The listing builds one solid part. Answer for the finished solid, in the listing's coordinates (mm). A direction names the side the tool comes from. Give positions to 0.01 mm unless a question says otherwise; leave off trailing zeros. Order: outer loops, then holes, each group sorted by start corner. A loop starts at its lowest first (then second) coordinate and runs counter-clockwise, first axis right, second up. Notation, with made-up numbers: (-12.5, -26) - (10.5, -26) arc R23 ccw to (10.5, 8) - close; hole circle Ø1 at (11.5, 17.25). An arc over 180 degrees is marked (long way). Use a Markdown table: item, result. Add a question column.
1) Find section C-C, the plane y = 0. Determine the outline of the cut face in (x, z).
2) Find section A-A, the plane x = -13.85. Determine the outline of the cut face in (y, z), plus the area to 3 significant figures.
3) Flat-ended cylindrical pins translate along their axes: pin 1 (1 mm diameter, centred on x = 10, z = 0.5, fed in from -Y); pin 2 (3 mm diameter, centred on x = -9, y = 0, fed in from +Z); pin 3 (0.6 mm diameter, centred on y = -12, z = 1.5, fed in from -X). Find the tip coordinate at first contact, or state that the pin passes through.
4) For faces 4 (the face through (12, -8.3, 1)), 5 (the face through (16, 0, 1)), 6 (the face through (0, 8.3, 1)), 7 (the face through (11.25, 0, 1)), 8 (the face through (-12, -8.3, 1)), determine the directions among +Z, -Z, +X, -X, +Y, -Y from which every point of the face is accessible in a straight line to the end or side of a thin tool.
5) The mould has two halves that part along Y. Classify faces 1 (the face through (7.5, -11, 1)), 2 (the face through (0, -13.55, 1)), 3 (the face through (0, -6.3, 1)): released by +Y, released by -Y, zero draft, split by the parting line, or undercut.
6) Straight lines are drawn through the part: line 1 (Y direction, x = 4.5, z = 1.25); line 2 (Y direction, x = 13.85, z = 0.85); line 3 (X direction, y = 0.25, z = 1.6). For each, find the intervals that lie inside material, in ascending order.
7) Find section D-D, the plane z = 0.85. Determine the outline of the cut face in (x, y), plus the area to 3 significant figures.
8) Find section B-B, the plane y = 4.75. Determine the outline of the cut face in (x, z), plus the area to 3 significant figures.
from build123d import *

# Parameters (mm, degrees)
SKETCH1_W           = 32
SKETCH1_H           = 16.6
SKETCH1_R           = 1
SKETCH1_W_2         = 22.5
SKETCH1_H_2         = 12.6
BOSS_EXTRUDE1_DEPTH = 2
SKETCH2_W           = 15
SKETCH2_H           = 2
BOSS_EXTRUDE2_DEPTH = 5.25


with BuildPart() as part:
    # Sketch1 → Boss-Extrude1 (new body)
    with BuildSketch(Plane.XY):
        Rectangle(SKETCH1_W, SKETCH1_H)
        with Locations((-13.85, 0)):
            Circle(SKETCH1_R, mode=Mode.SUBTRACT)
        with Locations((13.85, 0)):
            Circle(SKETCH1_R, mode=Mode.SUBTRACT)
        Rectangle(SKETCH1_W_2, SKETCH1_H_2, mode=Mode.SUBTRACT)
    extrude(amount=BOSS_EXTRUDE1_DEPTH)

    # Sketch2 → Boss-Extrude2 (add)
    with BuildSketch(Plane.XZ.offset(8.3)):
        with Locations((0, 1)):
            Rectangle(SKETCH2_W, SKETCH2_H)
    extrude(amount=BOSS_EXTRUDE2_DEPTH)


solid = part.part
The answers:
| question | item | result |
|---|---|---|
| 1 | outline | (-16, 0) - (-14.85, 0) - (-14.85, 2) - (-16, 2) - close; (-12.85, 0) - (-11.25, 0) - (-11.25, 2) - (-12.85, 2) - close; (11.25, 0) - (12.85, 0) - (12.85, 2) - (11.25, 2) - close; (14.85, 0) - (16, 0) - (16, 2) - (14.85, 2) - close |
| 2 | outline | (-8.3, 0) - (-1, 0) - (-1, 2) - (-8.3, 2) - close; (1, 0) - (8.3, 0) - (8.3, 2) - (1, 2) - close |
| 2 | area | 29.2 mm2 |
| 3 | pin 1 | y = -8.3 |
| 3 | pin 2 | through |
| 3 | pin 3 | x = -7.5 |
| 4 | face 4 | +Z, -Z, +X, -Y |
| 4 | face 5 | +Z, -Z, +X, +Y, -Y |
| 4 | face 6 | +Z, -Z, +X, -X, +Y |
| 4 | face 7 | +Z, -Z |
| 4 | face 8 | +Z, -Z, -X, -Y |
| 5 | face 1 | zero draft |
| 5 | face 2 | released by -Y |
| 5 | face 3 | undercut |
| 6 | line 1 | -13.55 to -6.3, 6.3 to 8.3 |
| 6 | line 2 | -8.3 to -1, 1 to 8.3 |
| 6 | line 3 | -16 to -14.82, -12.88 to -11.25, 11.25 to 12.88, 14.82 to 16 |
| 7 | outline | (-16, -8.3) - (-7.5, -8.3) - (-7.5, -13.55) - (7.5, -13.55) - (7.5, -8.3) - (16, -8.3) - (16, 8.3) - (-16, 8.3) - close; hole circle Ø2 at (-13.85, 0); hole (-11.25, -6.3) - (11.25, -6.3) - (11.25, 6.3) - (-11.25, 6.3) - close; hole circle Ø2 at (13.85, 0) |
| 7 | area | 320 mm2 |
| 8 | outline | (-16, 0) - (-11.25, 0) - (-11.25, 2) - (-16, 2) - close; (11.25, 0) - (16, 0) - (16, 2) - (11.25, 2) - close |
| 8 | area | 19.0 mm2 |
